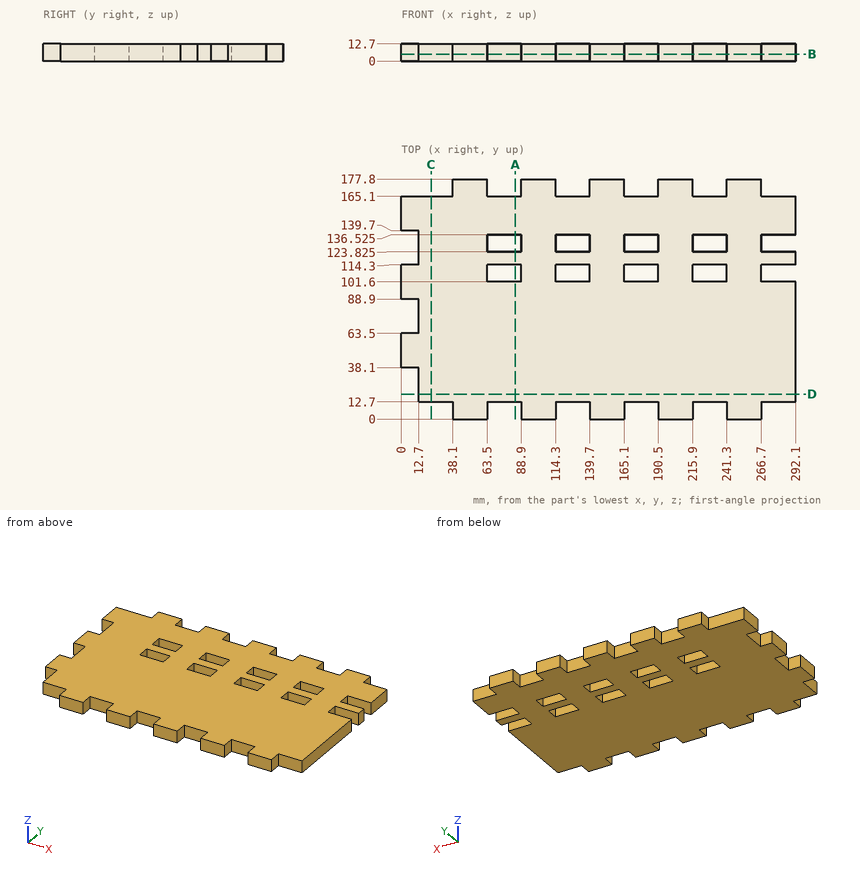
Source: three-view drawing plus pictorial views. Frame: mm from the lowest corner of the part. Give positions to 0.01 mm unless a question says otherwise; leave off trailing zeros. Order: outer loops, then holes, each group sorted by start corner. A loop starts at its lowest first (then second) coordinate and runs counter-clockwise, first axis right, second up.
1. Material intervals for L1, parallel to Y at x = 177.5, z = 7.25 (3 decimals); L2, parallel to X at y = 125, z = 11.25; L3, parallel to X at y = 113, z = 3.25, sorted ascending.
Derived:
L1: y = 12.7 to 101.6, 114.3 to 123.825, 136.525 to 165.1
L2: x = 12.7 to 63.5, 88.9 to 114.3, 139.7 to 165.1, 190.5 to 215.9, 241.3 to 266.7
L3: x = 0 to 63.5, 88.9 to 114.3, 139.7 to 165.1, 190.5 to 215.9, 241.3 to 266.7
2. Pin query (flat end, axial travel): pin 1 (12 mm diameter, centred on x = 199.5, y = 146.5, fed in from -Z); pin 2 (4 mm diameter, centred on x = 74, z = 9.5, fed in from -Y); pin 3 (4 mm diameter, centred on x = 178.5, z = 8, fed in from +Y); pin 4 (4 mm diameter, centred on y = 172, z = 4, fed in from -X). Return the tip coordinate at first contact, or that it passes through.
Derived:
pin 1: stops at z = 0
pin 2: stops at y = 12.7
pin 3: stops at y = 165.1
pin 4: stops at x = 38.1
3. Section C-C on x = 22. Return the cut outline in (y, z), and give its area (3 significant figures).
Derived:
outline: (12.7, 0) - (165.1, 0) - (165.1, 12.7) - (12.7, 12.7) - close
area: 1,940 mm2
4. Section B-B on z = 5.25. Give the number of separate pieces and of enclosed holes in the cut face, and give its area (3 significant figures).
Derived:
separate pieces: 1
enclosed holes: 8
area: 43,500 mm2
5. Section D-D on y = 18.5. Return the cut outline in (x, z).
Derived:
outline: (12.7, 0) - (292.1, 0) - (292.1, 12.7) - (12.7, 12.7) - close
6. Section A-A on x = 84.5. Return the cut outline in (y, z) (3 decimals).
Derived:
outline: (12.7, 0) - (101.6, 0) - (101.6, 12.7) - (12.7, 12.7) - close; (114.3, 0) - (123.825, 0) - (123.825, 12.7) - (114.3, 12.7) - close; (136.525, 0) - (165.1, 0) - (165.1, 12.7) - (136.525, 12.7) - close
